Autodesk Inventor part; units mm, degrees
ref_plane "YZ Plane" through (0, 0, 0) normal (1, 0, 0) x (0, 1, 0)
ref_plane "XZ Plane" through (0, 0, 0) normal (0, 1, 0) x (-1, 0, 0)
ref_plane "XY Plane" through (0, 0, 0) normal (0, 0, 1) x (1, 0, 0)
sketch "Sketch1" plane through (0, 0, 0) normal (0, 1, 0) x (-1, 0, 0)
  line L0 (0, 0) -> (0, -25.4)
  line L1 (0, -25.4) -> (1.5875, -25.4)
  line L2 (0, 0) -> (25.4, 0)
  line L3 (25.4, 0) -> (25.4, -1.5875)
  line L4 (25.4, -1.5875) -> (1.5875, -1.5875)
  line L5 (1.5875, -1.5875) -> (1.5875, -25.4)
  dimension "d0" = 25.4
  dimension "d1" = 1.5875
  dimension "d4" = 25.4
  dimension "d5" = 1.5875
extrude "Extrusion1" add sketch "Sketch1" along normal blind 114.3
sketch "Sketch2" plane through (-1.5875, 0, -25.4) normal (-1, 0, 0) x (0, 0, 1)
  circle A0 centre (-0.4334, 40.1699) radius 5.715
  point P0 (25.4, 0)
extrude "Extrusion2" cut sketch "Sketch2" against normal blind 46.0375
properties part number "OTHER bracket for pickup"
CAD build for the part. Positions are in the model's coordinates, mm. A direction names the side the tool comes from. Round coordinates to 2 decimals unless told otherwise and drop trailing zeros. Order: outer loops, then holes, each group sorted by start corner. A loop starts at its lowest first (then second) coordinate and runs counter-clockwise, first axis right, second up. Notation, with made-up numbers: (21.5, 66.25) - (77.5, 66.25) arc R29 cw to (77.5, 90.25) - close; hole circle Ø3 at (25, -30). An arc over 180 degrees is marked (long way). Answer in a Markdown table with one row per item. Add a question column.
(1) 3-axis set-ups, long thin cutter, end or side, ignore diameter. For faces 5 (the face through (-14, 56, -1.588)), 6 (the face through (-13, 56, 0)): which of +Z, -Z, +X, -X, +Y, -Y reach the whole face in a straight line?
(2) Band-saw the part on A-A on z = -22.25. List the corners of the cut face in (x, y).
(3) Band-saw the part on B-B on x = -15.75. List the corners of the cut face in (y, z).
(4) Drop flat-ended pins along their axis: pin 1 Ø1.5 at (y, z) = (60, -22) entering from -X; pin 2 Ø5 at (x, y) = (-14.5, 38) entering from -Z. Give the stop position or say it passes through.
(5) Band-saw the part on C-C on y = 82. List the corners of the cut face in (x, z), and give its area (3 significant figures).
(6) Mould opens along Y. For faces 1 (the face through (-1, 114.3, -7)), 2 (the face through (-1, 0, -7)), 3 (the face through (-0.8, 40.05, -20.12)), 4 (the face through (0, 56, -13)) say: +Y half, -Y half, draft (parallel to the pull), parting line (faces both ways), or undercut.
(7) Band-saw the part on D-D on z = -14.25. List the corners of the cut face in (x, y).
(8) Probe L1, parallel to Z at x = -8.5, y = 58.5. List the from-to ranges inside material, lowest first. Write a range as [from, to].
Data:
| question | item | result |
|---|---|---|
| 1 | face 5 | -Z, -X, +Y, -Y |
| 1 | face 6 | +Z, +X, -X, +Y, -Y |
| 2 | outline | (-1.59, 0) - (0, 0) - (0, 35.72) - (-1.59, 35.72) - close; (-1.59, 44.62) - (0, 44.62) - (0, 114.3) - (-1.59, 114.3) - close |
| 3 | outline | (0, -1.59) - (114.3, -1.59) - (114.3, 0) - (0, 0) - close |
| 4 | pin 1 | stops at x = -1.59 |
| 4 | pin 2 | stops at z = -1.59 |
| 5 | outline | (-25.4, -1.59) - (-1.59, -1.59) - (-1.59, -25.4) - (0, -25.4) - (0, 0) - (-25.4, 0) - close |
| 5 | area | 78.1 mm^2 |
| 6 | face 1 | +Y half |
| 6 | face 2 | -Y half |
| 6 | face 3 | undercut |
| 6 | face 4 | draft |
| 7 | outline | (-1.59, 0) - (0, 0) - (0, 114.3) - (-1.59, 114.3) - close |
| 8 | L1 | z = [-1.59, 0] |
